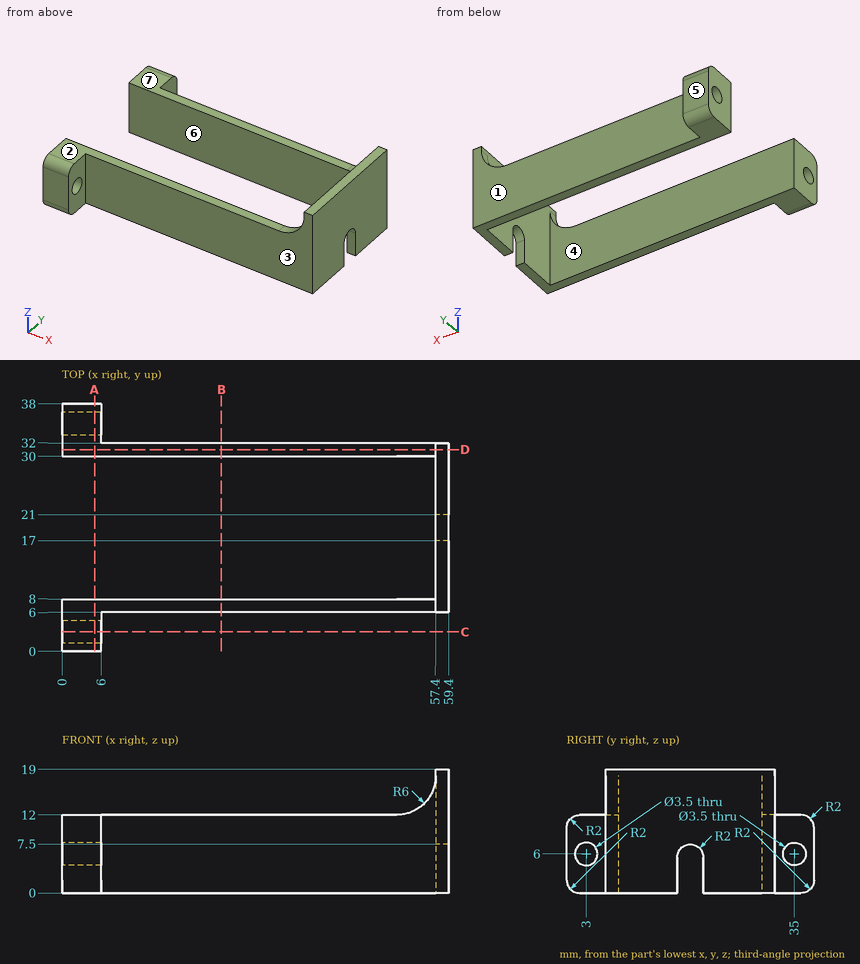
Print and shaded views of the part. All mm, measured from the part's lowest x, y and z. A direction names the side the tool comes from. Round coordinates to 2 decimals unless told otherwise and drop trailing zeros. Write each loop counter-clockwise with the first axis right and the second up, starting at its lowest first coordinate (ties: lowest second). Pieces come first, ordered by that corner, then holes. Notation, with made-up numbers: (8, -1) -> (24, -1) arc R23 ccw to (24, 13) -> close; hole circle Ø5 at (83, 15.25). An arc over 180 degrees is marked (long way). Return JSON: item names as keys, results as strings. Group by question number.
Q1. Saw through at D-D on y = 31. Write the cut outline in (x, z), plus the area to 3 significant figures.
Q2. Which spindle directions (+Z, -Z, +X, -X, +Y, -Y) get a long thin tool onto all of the face, cutting with end or side? Do the marked faces 1, 2, 3 and 4. Say none if no direction does.
Q3. Saw through at C-C on y = 3. Write the cut outline in (x, z), plus the area to 3 significant figures.
Q4. Probe L1, parallel to Y at x = 43, z = 5.75; L2, parallel to Y at x = 5.5, z = 5.75; L3, parallel to Z at x = 3, y = 3. List the from-to ranges inside material, lowest first. Write a range as [from, to].
Q5. Mould opens along Y. For the marked faces 5, 6 and 7 say: pulls with the +Y half, pulls with the -Y half, needs draft (parallel to the pull), parting line crosses it, or undercut.
Q6. Saw through at B-B on x = 24.5. Write the cut outline in (y, z), plus the area to 3 significant figures.
Q7. Saw through at A-A on x = 5. Write the cut outline in (y, z).
Q8. Pin check, flat tips, straight feed: pin 1 (1.5 mm diameter, centred on y = 5, z = 11.5, fed in from +X); pin 2 (5.5 mm diameter, centred on x = 30.5, z = 7, fed in from +Y); pin 3 (1.8 mm diameter, centred on x = 20, y = 32, fed in from +Z). Stop position of each tip, or through.
Answer:
{
 "1": {"outline": "(0, 0) -> (59.4, 0) -> (59.4, 19) -> (57.4, 19) -> (57.4, 18) arc R6 cw to (51.4, 12) -> (0, 12) -> close", "area": "735 mm2"},
 "2": {"face 1": "+Z, -Z, +X, +Y", "face 2": "+Z, -X, +Y, -Y", "face 3": "+Z, -Z, +X, -Y", "face 4": "+Z, -Z, -X"},
 "3": {"outline": "(0, 0) -> (6, 0) -> (6, 4.25) -> (0, 4.25) -> close; (0, 7.75) -> (6, 7.75) -> (6, 12) -> (0, 12) -> close", "area": "51.0 mm2"},
 "4": {"L1": "[6, 8], [30, 32]", "L2": "[0, 1.27], [4.73, 8], [30, 33.27], [36.73, 38]", "L3": "[0, 4.25], [7.75, 12]"},
 "5": {"face 5": "pulls with the +Y half", "face 6": "undercut", "face 7": "needs draft"},
 "6": {"outline": "(6, 0) -> (8, 0) -> (8, 12) -> (6, 12) -> close; (30, 0) -> (32, 0) -> (32, 12) -> (30, 12) -> close", "area": "48.0 mm2"},
 "7": {"outline": "(0, 2) arc R2 ccw to (2, 0) -> (8, 0) -> (8, 12) -> (2, 12) arc R2 ccw to (0, 10) -> close; (30, 0) -> (36, 0) arc R2 ccw to (38, 2) -> (38, 10) arc R2 ccw to (36, 12) -> (30, 12) -> close; hole circle Ø3.5 at (3, 6); hole circle Ø3.5 at (35, 6)"},
 "8": {"pin 1": "x = 6", "pin 2": "y = 32", "pin 3": "z = 12"}
}
